Verification items for the finished model (mm, model axes). A direction names the side the tool comes from. Give positions to 0.01 mm unless a question says otherwise; leave off trailing zeros. One line per item, written item: value. Start each with the question number.
1. Gauge pin test, flat ends, axial feed: pin 1 (6.5 mm diameter, centred on x = 1.5, y = 7, fed in from +Z); pin 2 (2 mm diameter, centred on y = -9.5, z = 16.5, fed in from -X); pin 3 (1 mm diameter, centred on y = -10.5, z = 77.5, fed in from +X); pin 4 (3 mm diameter, centred on x = 2.5, z = -38, fed in from -Y). Record the tip position at first contact, or that the pin passes through.
2. Mould release check, pull along Z, two halves, no side actions. Record for faces 4 (the cylindrical face through (-26.36, 17.46, -5.85)), 5 (the flat face through (-12, 20, 12)), 6 (the flat face through (-42.756, 0.14, -24.685)): pulls with the +Z half, pulls with the -Z half, needs draft (parallel to the pull), parting line crosses it, or undercut.
3. Access from +Z, -Z, +X, -X, +Y, -Y to the whole of each face (thin tool, end or side, straight path). Record for faces 1 (the flat face through (20.2, -10, -25.1)), 2 (the flat face through (-42.52, 0.14, 24.55)), 3 (the conical face through (-80.546, -5.041, -10.575)).
4. Sectioned sample at A-A (x = 0). Count the separate pieces of the cut face and the enclosed holes in it, plus the area to 3 significant figures.
5. Scan lines: L1, parallel to X at y = -14.95, z = 0; L2, parallel to Z at x = 29, y = -2.5; L3, parallel to X at y = 11, z = -8. Record each from-to range of solid material in increasing order. Write a range as [from, to].
from build123d import *

# Parameters (mm, degrees)
SKETCH1_R                 = 100
BOSS_EXTRUDE1_DEPTH       = 10
BOSS_EXTRUDE3_DEPTH       = 10
BOSS_EXTRUDE3_DEPTH_BACK  = 30
SKETCH2_R                 = 27
SKETCH4_R                 = 27
BOSS_EXTRUDE4_DEPTH       = 5
BOSS_EXTRUDE11_DEPTH      = 5
BOSS_EXTRUDE11_DEPTH_BACK = 25
SKETCH7_R                 = 100
SKETCH7_R_2               = 72
CUT_EXTRUDE1_DEPTH        = 147.969384567
FILLET1_R                 = 5
FILLET2_R                 = 5


with BuildPart() as part:
    # Sketch1 → Boss-Extrude1 (new, symmetric)
    with BuildSketch(Plane(origin=(0, 0, 0), x_dir=(1, 0, 0), z_dir=(0, 1, 0))):
        with Locations(Location((0, 0, 0), (0, 0, 270))):
            Circle(SKETCH1_R)
        with BuildLine():
            Line((-17.5, 30.310889132), (-32, 55.425625842))
            ThreePointArc((-32, 55.425625842), (0, 64), (32, 55.425625842))
            Line((32, 55.425625842), (17.5, 30.310889132))
            ThreePointArc((17.5, 30.310889132), (0, 35), (-17.5, 30.310889132))
        make_face(mode=Mode.SUBTRACT)
        with BuildLine():
            Line((30.310889132, 17.5), (55.425625842, 32))
            ThreePointArc((55.425625842, 32), (64, 0), (55.425625842, -32))
            Line((55.425625842, -32), (30.310889132, -17.5))
            ThreePointArc((30.310889132, -17.5), (35, 0), (30.310889132, 17.5))
        make_face(mode=Mode.SUBTRACT)
        with BuildLine():
            Line((17.5, -30.310889132), (32, -55.425625842))
            ThreePointArc((32, -55.425625842), (0, -64), (-32, -55.425625842))
            Line((-32, -55.425625842), (-17.5, -30.310889132))
            ThreePointArc((-17.5, -30.310889132), (0, -35), (17.5, -30.310889132))
        make_face(mode=Mode.SUBTRACT)
        with BuildLine():
            Line((-30.310889132, -17.5), (-55.425625842, -32))
            ThreePointArc((-55.425625842, -32), (-64, 0), (-55.425625842, 32))
            Line((-55.425625842, 32), (-30.310889132, 17.5))
            ThreePointArc((-30.310889132, 17.5), (-35, 0), (-30.310889132, -17.5))
        make_face(mode=Mode.SUBTRACT)
    extrude(amount=BOSS_EXTRUDE1_DEPTH, both=True)

    # Sketch2 → Boss-Extrude3 (add, two sides: drawn at the far end of the back side and taken through both)
    with BuildSketch(Plane(origin=(0, 10, 0), x_dir=(1, 0, 0), z_dir=(0, 1, 0)).offset(-BOSS_EXTRUDE3_DEPTH_BACK)):
        with Locations(Location((0, 0, 0), (0, 0, 270))):
            Circle(SKETCH2_R)
    extrude(amount=BOSS_EXTRUDE3_DEPTH + BOSS_EXTRUDE3_DEPTH_BACK)

    # Sketch4 → Boss-Extrude4 (add, symmetric)
    with BuildSketch(Plane.XZ.offset(10)):
        with Locations(Location((0, 0, 0), (0, 0, 90))):
            Circle(SKETCH4_R)
    extrude(amount=BOSS_EXTRUDE4_DEPTH, both=True)

    # Sketch7 → Boss-Extrude11 (add, two sides: drawn at the far end of the back side and taken through both)
    with BuildSketch(Plane.XZ.offset(10).offset(-BOSS_EXTRUDE11_DEPTH_BACK)):
        with Locations(Location((0, 0, 0), (0, 0, 270))):
            Circle(SKETCH7_R)
        with Locations(Location((0, 0, 0), (0, 0, 270))):
            Circle(SKETCH7_R_2, mode=Mode.SUBTRACT)
    extrude(amount=BOSS_EXTRUDE11_DEPTH + BOSS_EXTRUDE11_DEPTH_BACK)

    # Sketch8 → Cut-Extrude1 (cut, through all)
    with BuildSketch(Plane(origin=(0, 20, 0), x_dir=(1, 0, 0), z_dir=(0, 1, 0))):
        with BuildLine():
            Line((-4, 14.456832295), (-4, 18.762826765))
            Line((-4, 18.762826765), (4, 18.762826765))
            Line((4, 18.762826765), (4, 14.456832295))
            ThreePointArc((4, 14.456832295), (7.5, 12.990381057), (10.519984026, 10.692517763))
            Line((10.519984026, 10.692517763), (14.249084625, 12.845514997))
            Line((14.249084625, 12.845514997), (18.249084625, 5.917311767))
            Line((18.249084625, 5.917311767), (14.519984026, 3.764314532))
            ThreePointArc((14.519984026, 3.764314532), (15, 0), (14.519984026, -3.764314532))
            Line((14.519984026, -3.764314532), (18.249084625, -5.917311767))
            Line((18.249084625, -5.917311767), (14.249084625, -12.845514997))
            Line((14.249084625, -12.845514997), (10.519984026, -10.692517763))
            ThreePointArc((10.519984026, -10.692517763), (7.5, -12.990381057), (4, -14.456832295))
            Line((4, -14.456832295), (4, -18.762826765))
            Line((4, -18.762826765), (-4, -18.762826765))
            Line((-4, -18.762826765), (-4, -14.456832295))
            ThreePointArc((-4, -14.456832295), (-7.5, -12.990381057), (-10.519984026, -10.692517763))
            Line((-10.519984026, -10.692517763), (-14.249084625, -12.845514997))
            Line((-14.249084625, -12.845514997), (-18.249084625, -5.917311767))
            Line((-18.249084625, -5.917311767), (-14.519984026, -3.764314532))
            ThreePointArc((-14.519984026, -3.764314532), (-15, 0), (-14.519984026, 3.764314532))
            Line((-14.519984026, 3.764314532), (-18.249084625, 5.917311767))
            Line((-18.249084625, 5.917311767), (-14.249084625, 12.845514997))
            Line((-14.249084625, 12.845514997), (-10.519984026, 10.692517763))
            ThreePointArc((-10.519984026, 10.692517763), (-7.5, 12.990381057), (-4, 14.456832295))
        make_face()
    extrude(amount=-CUT_EXTRUDE1_DEPTH, mode=Mode.SUBTRACT)

    # Sketch9 → Cut-Revolve4 (revolve, cut)
    with BuildSketch(Plane(origin=(0, 0, 0), x_dir=(0, 0, -1), z_dir=(1, 0, 0))):
        Polygon((-80, 4.71), (-80, -4.71), (-99.775475202, -10.00882261), (-116.246670556, -10.00882261), (-116.246670556, 9.978109538), (-99.839422916, 9.978109538), (-99.775475202, 10.00882261), align=None)
    revolve(axis=Axis((0, 78.143519102, 0), (0, -1, 0)), mode=Mode.SUBTRACT)

    # Fillet1
    fillet1_edges = [part.edges().sort_by_distance(p)[0] for p in [
        (0, 10, -27),
        (0, -10, -27),
        (0, -10, 72),
        (0, 10, 72),
    ]]
    fillet(fillet1_edges, radius=FILLET1_R - 0.0001)  # a hair under: the kernel refuses the full size

    # Fillet2
    fillet2_edges = [part.edges().sort_by_distance(p)[0] for p in [
        (30.310889132, 0, -17.5),
        (30.310889132, 0, 17.5),
        (55.425625842, 0, 32),
        (55.425625842, 0, -32),
        (17.5, 0, 30.310889132),
        (-17.5, 0, 30.310889132),
        (-32, 0, 55.425625842),
        (32, 0, 55.425625842),
        (-30.310889132, 0, 17.5),
        (-30.310889132, 0, -17.5),
        (-55.425625842, 0, -32),
        (-55.425625842, 0, 32),
        (-17.5, 0, -30.310889132),
        (17.5, 0, -30.310889132),
        (32, 0, -55.425625842),
        (-32, 0, -55.425625842),
    ]]
    fillet(fillet2_edges, radius=FILLET2_R)


solid = part.part
Results are:
1. pin 1: stops at z = 100
1. pin 2: stops at x = -98.77
1. pin 3: stops at x = 63.8
1. pin 4: passes through
2. face 4: parting line crosses it
2. face 5: needs draft
2. face 6: undercut
3. face 1: -Y
3. face 2: +Y, -Y
3. face 3: none
4. separate pieces: 4
4. enclosed holes: 0
4. area: 2,430 mm^2
5. L1: x = [-100, -72], [-27, -15], [15, 27], [72, 100]
5. L2: z = [-74.56, -56.49], [-50.23, 50.23], [56.49, 74.56]
5. L3: x = [-99.68, -69.54], [-27.87, -17.05], [17.05, 27.87], [69.54, 99.68]
